Geometry check sheet. Reference: the model listing, model coordinates, mm. A direction names the side the tool comes from. Coordinates: 2 decimals unless noted, no trailing zeros. Write each loop counter-clockwise with the first axis right and the second up, starting at its lowest first coordinate (ties: lowest second). Pieces come first, ordered by that corner, then holes. Notation, with made-up numbers: (66, 40.5) -> (110, 40.5) arc R9 cw to (110, 51.5) -> close; hole circle Ø8 at (-9.75, -4.5). An arc over 180 degrees is marked (long way). Use a Markdown table: item, result.
```python
from build123d import *

# Parameters (mm, degrees)
SKETCH1_W             = 12.7
SKETCH1_H             = 5.08
BOSS_EXTRUDE1_DEPTH   = 10.16
SKETCH2_W             = 12.7
SKETCH2_H             = 0.762
BOSS_EXTRUDE3_DEPTH   = 3.81
BOSS_EXTRUDE4_DEPTH   = 3.81
BODY_MOVE_COPY3_ANGLE = 90
BODY_MOVE_COPY6_ANGLE = 180
BOSS_EXTRUDE6_DEPTH   = 10.16
SKETCH17_W            = 12.7
SKETCH17_H            = 0.586972929
SKETCH17_H_2          = 0.560182851
SKETCH17_H_3          = 0.470375136
SKETCH17_W_2          = 0.38891101
SKETCH17_H_4          = 12.7
SKETCH17_W_3          = 0.566388334
SKETCH17_W_4          = 0.460759313
SKETCH17_W_5          = 0.522714126
SKETCH17_W_6          = 0.418299814
SKETCH17_W_7          = 0.466316337
SKETCH17_H_5          = 12.693652269
BOSS_EXTRUDE10_DEPTH  = 0.127
SKETCH18_W            = 0.762
SKETCH18_H            = 12.7
SKETCH18_W_2          = 12.7
SKETCH18_H_2          = 0.762
BOSS_EXTRUDE11_DEPTH  = 2.54


with BuildPart() as part:
    # Sketch1 → Boss-Extrude1 (new body)
    with BuildSketch(Plane.XY):
        with Locations((6.35, 2.54)):
            Rectangle(SKETCH1_W, SKETCH1_H)
    extrude(amount=BOSS_EXTRUDE1_DEPTH)

    # Sketch2 → Boss-Extrude3 (add)
    with BuildSketch(Plane(origin=(0, 5.08, 0), x_dir=(1, 0, 0), z_dir=(0, 1, 0))):
        with Locations((6.35, -0.381)):
            Rectangle(SKETCH2_W, SKETCH2_H)
    extrude(amount=BOSS_EXTRUDE3_DEPTH)

    # Sketch4 → Boss-Extrude4 (add)
    with BuildSketch(Plane(origin=(0, 5.08, 0), x_dir=(1, 0, 0), z_dir=(0, 1, 0))):
        Polygon((1.196042578, -2.061016669), (0, -2.061016669), (0, -1.299016669), (1.196042578, -1.299016669), (12.7, -1.299016669), (12.7, -2.061016669), align=None)
    extrude(amount=BOSS_EXTRUDE4_DEPTH)


with BuildPart() as body_2:
    # Body-Move/Copy1: copy of part
    add(part.part.moved(Location((-19.746027861, 19.169390197, 0))))


with BuildPart() as body_2_1:
    # Body-Move/Copy3: moved
    add(body_2.part.rotate(Axis((-13.396027861, 25.765927537, 0), (0, 0, -1)), BODY_MOVE_COPY3_ANGLE))


with BuildPart() as body_3:
    # Body-Move/Copy5: copy of body 2
    add(body_2_1.part.moved(Location((40.507721278, -2.230163532, 0))))


with BuildPart() as body_3_1:
    # Body-Move/Copy6: moved
    add(body_3.part.rotate(Axis((27.111693417, 25.765927537, 0), (0, 0, 1)), BODY_MOVE_COPY6_ANGLE))


with BuildPart() as body_3_2:
    # Body-Move/Copy7: moved
    add(body_3_1.part.moved(Location((-7.419705442, -9.040319303, 0))))


with BuildPart() as body_2_2:
    # Body-Move/Copy8: moved
    add(body_2_1.part.moved(Location((5.274716885, -2.873342861, 0))))


with BuildPart() as part_1:
    add(part.part)

    add(body_2_2.part)  # Boss-Extrude6 merges body 2

    add(body_3_2.part)  # Boss-Extrude6 merges body 3
    # Sketch12 → Boss-Extrude6 (add)
    with BuildSketch(Plane.XY.offset(10.16)):
        with BuildLine():
            Line((-14.717848316, 16.542584676), (-13.364641255, 16.542584676))
            ThreePointArc((-13.364641255, 16.542584676), (-9.804171486, 6.237862161), (0, 1.46895531))
            Line((0, 1.46895531), (0, 0))
            ThreePointArc((0, 0), (-10.785005623, 5.223126147), (-14.717848316, 16.542584676))
        make_face()
        with BuildLine():
            Line((12.7, 1.46895531), (12.7, 0))
            ThreePointArc((12.7, 0), (22.105003473, 3.488610144), (26.288525315, 12.605771766))
            Line((26.288525315, 12.605771766), (24.975782085, 12.605771766))
            ThreePointArc((24.975782085, 12.605771766), (21.144401251, 4.494965824), (12.7, 1.46895531))
        make_face()
    extrude(amount=-BOSS_EXTRUDE6_DEPTH)

    # Sketch17 → Boss-Extrude10 (add)
    with BuildSketch(Plane.XY.offset(0.762)):
        with Locations((6.35, 8.007004569)):
            Rectangle(SKETCH17_W, SKETCH17_H)
        with Locations((6.35, 6.9171208)):
            Rectangle(SKETCH17_W, SKETCH17_H_2)
        with Locations((6.35, 5.881481875)):
            Rectangle(SKETCH17_W, SKETCH17_H_3)
        with Locations((-6.478997016, 22.892584676)):
            Rectangle(SKETCH17_W_2, SKETCH17_H_4)
        with Locations((-7.666574601, 22.892584676)):
            Rectangle(SKETCH17_W_3, SKETCH17_H_4)
        with Locations((-8.807561086, 22.892584676)):
            Rectangle(SKETCH17_W_4, SKETCH17_H_4)
        with Locations((20.31529367, 18.955771766)):
            Rectangle(SKETCH17_W_5, SKETCH17_H_4)
        with Locations((19.241203682, 18.955771766)):
            Rectangle(SKETCH17_W_6, SKETCH17_H_4)
        with Locations((18.30794503, 18.958945632)):
            Rectangle(SKETCH17_W_7, SKETCH17_H_5)
    extrude(amount=BOSS_EXTRUDE10_DEPTH)

    # Sketch18 → Boss-Extrude11 (add)
    with BuildSketch(Plane.XY.offset(2.061016669)):
        with Locations((-9.256848316, 22.892584676)):
            Rectangle(SKETCH18_W, SKETCH18_H)
        with Locations((6.35, 5.461)):
            Rectangle(SKETCH18_W_2, SKETCH18_H_2)
        with Locations((20.827525315, 18.955771766)):
            Rectangle(SKETCH18_W, SKETCH18_H)
    extrude(amount=BOSS_EXTRUDE11_DEPTH)


solid = part_1.part
```
Item 1: Tool access check on faces 1 (the flat face through (-10, 16.543, 4)), 2 (the flat face through (12.7, 4, 4)), 3 (the flat face through (6, 7, 2.061)), 4 (the flat face through (23, 25.306, 4)). Record the directions out of +Z, -Z, +X, -X, +Y, -Y that give a thin tool (end or side, any length) a straight path to the whole face; none if there is none.
Answer block:
| item | result |
|---|---|
| face 1 | +Z, -Z |
| face 2 | +Z, -Z, +Y |
| face 3 | +Z, +Y |
| face 4 | +Z, -Z, +X, +Y |
Item 2: Section check A-A on z = 3. Record the boundary of the cut face in (x, y).
Answer block:
| item | result |
|---|---|
| outline | (-14.72, 16.54) arc R15.66 ccw to (0, 0) -> (12.7, 0) arc R13.11 ccw to (26.29, 12.61) -> (26.29, 25.31) -> (20.45, 25.31) -> (20.45, 12.61) -> (24.98, 12.61) arc R11.72 cw to (12.7, 1.47) -> (12.7, 5.84) -> (0, 5.84) -> (0, 1.47) arc R14.24 cw to (-13.36, 16.54) -> (-8.88, 16.54) -> (-8.88, 29.24) -> (-14.72, 29.24) -> close |
Item 3: Section check D-D on x = 24.5. Record the boundary of the cut face in (y, z).
Answer block:
| item | result |
|---|---|
| outline | (6.47, 0) -> (9.82, 0) -> (9.82, 10.16) -> (6.47, 10.16) -> close; (12.61, 0) -> (25.31, 0) -> (25.31, 10.16) -> (12.61, 10.16) -> close |
Item 4: Section check C-C on y = 4. Record the boundary of the cut face in (x, z), then the cut area to 3 significant figures.
Answer block:
| item | result |
|---|---|
| outline | (-9.57, 0) -> (-7.29, 0) -> (-7.29, 10.16) -> (-9.57, 10.16) -> close; (0, 0) -> (12.7, 0) -> (12.7, 10.16) -> (0, 10.16) -> close; (20.56, 0) -> (22.63, 0) -> (22.63, 10.16) -> (20.56, 10.16) -> close |
| area | 173 mm^2 |
Item 5: Section check B-B on x = 5.5. Record the boundary of the cut face in (y, z).
Answer block:
| item | result |
|---|---|
| outline | (0, 0) -> (8.89, 0) -> (8.89, 0.76) -> (8.3, 0.76) -> (8.3, 0.89) -> (7.71, 0.89) -> (7.71, 0.76) -> (7.2, 0.76) -> (7.2, 0.89) -> (6.64, 0.89) -> (6.64, 0.76) -> (6.12, 0.76) -> (6.12, 0.89) -> (5.65, 0.89) -> (5.65, 0.76) -> (5.08, 0.76) -> (5.08, 1.3) -> (8.89, 1.3) -> (8.89, 2.06) -> (5.84, 2.06) -> (5.84, 4.6) -> (5.08, 4.6) -> (5.08, 10.16) -> (0, 10.16) -> close |
Item 6: Thickness scan on L1, parallel to Z at x = 21, y = 17.5; L2, parallel to X at y = 5, z = 6.5; L3, parallel to X at y = 19.25, z = 8.5. Record the ranges inside material, lowest first. Write a range as [from, to].
Answer block:
| item | result |
|---|---|
| L1 | z = [0, 0.76], [1.3, 4.6] |
| L2 | x = [-10.58, -8.56], [0, 12.7], [21.67, 23.5] |
| L3 | x = [-14.72, -9.64], [21.21, 26.29] |
Item 7: Depth check by flat-ended pin: P1, Ø6, axis at x = 15.5, z = 6.5, coming from the +Y side; P2, Ø3, axis at x = 9, z = 3, coming from the +Y side; P3, Ø1, axis at x = 5, z = 7.5, coming from the -Y side. Enter the tip coordinate at first touch or a pass-through.
Answer block:
| item | result |
|---|---|
| P1 | stops at y = 5.08 |
| P2 | stops at y = 8.89 |
| P3 | stops at y = 0 |
Item 8: Mould release check, pull along X, two halves, no side actions. Record for faces 5 (the flat face through (26.289, 19, 5)), 6 (the flat face through (-8.876, 23, 3)), 7 (the flat face through (6, 8, 0)): +X half, -X half, draft (parallel to the pull), parting line (faces both ways), or undercut.
Answer block:
| item | result |
|---|---|
| face 5 | +X half |
| face 6 | undercut |
| face 7 | draft |
